```python
from build123d import *

# Parameters (mm, degrees)
F0_W     = 558.8
F0_H     = 31.75
F1_DEPTH = 31.75


with BuildPart() as f1:
    # F0 (on Front) → F1 (new body)
    with BuildSketch(Plane.XZ):
        Polygon((0, 711.2), (0, 0), (31.75, 0), (31.75, 95.25), (31.75, 127), (31.75, 920.75), (31.75, 952.5), (31.75, 1357.598856), (279.4, 1165.543754), (279.4, 952.5), (311.15, 952.5), (311.15, 1181.1), (0, 1422.4), (0, 952.5), align=None)
        Polygon((590.55, 127), (590.55, 95.25), (590.55, 0), (622.3, 0), (622.3, 711.2), (311.15, 952.5), (279.4, 952.5), (31.75, 952.5), (31.75, 920.75), (300.28142, 920.75), (590.55, 695.643754), align=None)
        with Locations((311.15, 111.125)):
            Rectangle(F0_W, F0_H)
    extrude(amount=F1_DEPTH)


solid = f1.part
```
Check sheet for the modelled part. Datum: model origin and axes. Units: mm. A direction names the side the tool comes from. Round coordinates to 2 decimals unless told otherwise and drop trailing zeros. Order: outer loops, then holes, each group sorted by start corner. A loop starts at its lowest first (then second) coordinate and runs counter-clockwise, first axis right, second up. Notation, with made-up numbers: (37.25, 74) - (74.25, 74) arc R17 cw to (74.25, 103) - close; hole circle Ø4 at (57.5, -33.75). An arc over 180 degrees is marked (long way). Write item = value, one per line.
Q1. Section check A-A (z = 509.5). Record the boundary of the cut face in (x, y), and give its area (3 significant figures).
Computed:
outline = (0, -31.75) - (31.75, -31.75) - (31.75, 0) - (0, 0) - close; (590.55, -31.75) - (622.3, -31.75) - (622.3, 0) - (590.55, 0) - close
area = 2,020 mm^2
Q2. Section check B-B (x = 216.5). Record the boundary of the cut face in (y, z), and give its area (3 significant figures).
Computed:
outline = (-31.75, 95.25) - (0, 95.25) - (0, 127) - (-31.75, 127) - close; (-31.75, 920.75) - (0, 920.75) - (0, 952.5) - (-31.75, 952.5) - close; (-31.75, 1214.32) - (0, 1214.32) - (0, 1254.5) - (-31.75, 1254.5) - close
area = 3,290 mm^2
Q3. Section check C-C (y = -26). Record the boundary of the cut face in (x, z), and give its area (3 significant figures).
Computed:
outline = (0, 0) - (31.75, 0) - (31.75, 95.25) - (590.55, 95.25) - (590.55, 0) - (622.3, 0) - (622.3, 711.2) - (311.15, 952.5) - (311.15, 1181.1) - (0, 1422.4) - close; hole (31.75, 127) - (590.55, 127) - (590.55, 695.64) - (300.28, 920.75) - (31.75, 920.75) - close; hole (31.75, 952.5) - (279.4, 952.5) - (279.4, 1165.54) - (31.75, 1357.6) - close
area = 123,000 mm^2
Q4. Tool access check on faces 4 (the face through (311.15, -16, 1065)), 5 (the face through (0, -16, 721)), 6 (the face through (279.4, -16, 1061)), 7 (the face through (307, -16, 95.25)). Record the directions out of +Z, -Z, +X, -X, +Y, -Y that give a thin tool (end or side, any length) a straight path to the whole face; none if there is none.
Computed:
face_4 = +Z, +X, +Y, -Y
face_5 = +Z, -Z, -X, +Y, -Y
face_6 = +Y, -Y
face_7 = -Z, +Y, -Y
Q5. Section check D-D (x = 435.5). Record the boundary of the cut face in (y, z).
Computed:
outline = (-31.75, 95.25) - (0, 95.25) - (0, 127) - (-31.75, 127) - close; (-31.75, 815.89) - (0, 815.89) - (0, 856.07) - (-31.75, 856.07) - close
Q6. Thickness scan on line 1 along X through (y, z) = (-18, 961); line 2 along X through (y, z) = (-1.5, 675); line 3 along Z through (x, y) = (105.5, -10.5). Record the ranges inside material, lowest first.
Computed:
line_1 = 0 to 31.75, 279.4 to 311.15
line_2 = 0 to 31.75, 590.55 to 622.3
line_3 = 95.25 to 127, 920.75 to 952.5, 1300.4 to 1340.58
Q7. Go/stop test with flat-tipped pins: pin 1 (12 mm diameter, centred on x = 394, z = 836, fed in from -Y) (1 decimal); pin 2 (10 mm diameter, centred on x = 550, y = -21, fed in from -Z); pin 3 (10 mm diameter, centred on x = 302, y = -28, fed in from +Z); pin 4 (9.5 mm diameter, centred on y = -20, z = 1012, fed in from +X). Record where each tip stops, or that it passes through.
Computed:
pin_1 = through
pin_2 = 95.25
pin_3 = 1192.07
pin_4 = 311.15
Q8. Draft check along X on faces 1 (the face through (606, -16, 0)), 2 (the face through (468.903, -15.653, 830.161)), 3 (the face through (31.75, -16, 47)). Enter one of: pulls with the +X half, pulls with the -X half, needs draft (parallel to the pull), parting line crosses it, or undercut.
Computed:
face_1 = needs draft
face_2 = pulls with the +X half
face_3 = undercut
